```python
from build123d import *

# Parameters (mm, degrees)
F1_DEPTH = 25
F2_T     = -2.5
F3_R     = 6.1653631348
F3_R_2   = 3.2347943308
F3_R_3   = 5.0463552764
F4_DEPTH = 25


with BuildPart() as f1:
    # F0 (on Top) → F1 (new body)
    with BuildSketch(Plane.XY):
        with BuildLine():
            Line((-20.0959555805, 59.7160309553), (-20.0959555805, 10.4758823072))
            ThreePointArc((-20.0959555805, 10.4758823072), (-0.1794521824, -22.6618476237), (20.2593356371, 10.1563212016))
            Line((20.2593356371, 10.1563212016), (20.2593356371, 59.7160309553))
            Line((20.2593356371, 59.7160309553), (-20.0959555805, 59.7160309553))
        make_face()
    extrude(amount=F1_DEPTH)

    # F2
    f2_openings = [f1.faces().sort_by_distance(p)[0] for p in [
        (0.050089, 19.786253, 25),
    ]]
    offset(amount=F2_T, openings=f2_openings, kind=Kind.INTERSECTION)

    # F3 (on face) → F4 (cut)
    with BuildSketch(Plane(origin=(-20.0959555805, 0, 0), x_dir=(0, -1, 0), z_dir=(-1, 0, 0))):
        with Locations((-48.8511435688, 13.3156133816)):
            Circle(F3_R)
        with Locations((-33.0031141639, 13.3156133816)):
            Circle(F3_R_2)
        with Locations((-20.0959555805, 13.3156133816)):
            Circle(F3_R_3)
    extrude(amount=-F4_DEPTH, mode=Mode.SUBTRACT)


solid = f1.part
```
Geometry check sheet. Reference: the model listing, model coordinates, mm. A direction names the side the tool comes from. Coordinates: 2 decimals unless noted, no trailing zeros. Order: outer loops, then holes, each group sorted by start corner. A loop starts at its lowest first (then second) coordinate and runs counter-clockwise, first axis right, second up. Notation, with made-up numbers: (87.5, -14.75) - (134.5, -14.75) arc R10 cw to (134.5, -4.75) - close; hole circle Ø4 at (53, -39.75). An arc over 180 degrees is marked (long way). Answer as a JSON object with one key per item and string values. Group by question number.
Item 1: Tool access check on faces 5 (the face through (-18.86, 55.01, 13.59)), 6 (the face through (0, 57.216, 14)), 7 (the face through (20.259, 35, 12)), 8 (the face through (-0.828, -22.647, 12.325)), 9 (the face through (-20.096, 35, 10)). Record the directions out of +Z, -Z, +X, -X, +Y, -Y that give a thin tool (end or side, any length) a straight path to the whole face; none if there is none.
Item 2: Depth check by flat-ended pin: pin 1 Ø4 at (y, z) = (33, 13.32) entering from +X; pin 2 Ø11 at (y, z) = (48.85, 13.32) entering from -X; pin 3 Ø5 at (y, z) = (-7.5, 12) entering from +X. Enter the tip coordinate at first touch or a pass-through.
Item 3: Sectioned sample at A-A, the plane z = 5.25. Record the cut outline in (x, y).
Item 4: Scan lines: probe 1 along X at (y, z) = (17, 6); probe 2 along Y at (x, z) = (0, 13.75); probe 3 along Z at (x, y) = (-10, 3). Record each from-to range of solid material in increasing order.
Item 5: Sectioned sample at B-B, the plane y = 53.5. Record the cut outline in (x, z), and give its area (3 significant figures).
Item 6: Draft check along Z on faces 1 (the face through (-18.863, 30.015, 12.077)), 2 (the face through (18, 19, 25)), 3 (the face through (-18.86, 17.38, 17.57)), 4 (the face through (-0.75, -20.15, 13.59)). Enter one of: +Z half, -Z half, draft (parallel to the pull), parting line (faces both ways), or undercut.
Item 7: Sectioned sample at C-C, the plane x = 0. Record the cut outline in (y, z).
Item 8: Sectioned sample at D-D, the plane z = 11.75. Record the cut outline in (x, y), and give its area (3 significant figures).
Resolved:
{
 "1": {"face 5": "-X", "face 6": "+Z", "face 7": "+Z, -Z, +X, +Y", "face 8": "+Z, -Z", "face 9": "+Z, -Z, -X, +Y"},
 "2": {"pin 1": "x = 20.26", "pin 2": "x = 17.76", "pin 3": "x = 22.1"},
 "3": {"outline": "(-20.1, 10.48) arc R22.66 ccw (long way) to (20.26, 10.16) - (20.26, 59.72) - (-20.1, 59.72) - close; hole (-17.6, 9.84) arc R20.16 ccw (long way) to (17.76, 9.55) - (17.76, 57.22) - (-17.6, 57.22) - close"},
 "4": {"probe 1": "-20.1 to -17.6, 17.76 to 20.26", "probe 2": "-22.66 to -20.16, 57.22 to 59.72", "probe 3": "0 to 2.5"},
 "5": {"outline": "(-20.1, 0) - (20.26, 0) - (20.26, 25) - (17.76, 25) - (17.76, 2.5) - (-17.6, 2.5) - (-17.6, 9.27) - (-20.1, 9.27) - close; (-20.1, 17.37) - (-17.6, 17.37) - (-17.6, 25) - (-20.1, 25) - close", "area": "193 mm^2"},
 "6": {"face 1": "undercut", "face 2": "+Z half", "face 3": "undercut", "face 4": "draft"},
 "7": {"outline": "(-22.66, 0) - (59.72, 0) - (59.72, 25) - (57.22, 25) - (57.22, 2.5) - (-20.16, 2.5) - (-20.16, 25) - (-22.66, 25) - close"},
 "8": {"outline": "(-20.1, 10.48) arc R22.66 ccw (long way) to (20.26, 10.16) - (20.26, 59.72) - (-20.1, 59.72) - (-20.1, 54.81) - (-17.6, 54.81) - (-17.6, 57.22) - (17.76, 57.22) - (17.76, 9.55) arc R20.16 cw (long way) to (-17.6, 9.84) - (-17.6, 15.3) - (-20.1, 15.3) - close; (-20.1, 24.89) - (-17.6, 24.89) - (-17.6, 30.17) - (-20.1, 30.17) - close; (-20.1, 35.83) - (-17.6, 35.83) - (-17.6, 42.89) - (-20.1, 42.89) - close", "area": "489 mm^2"}
}
